```python
from build123d import *

# Parameters (mm, degrees)
SKETCH2_W           = 31.88
SKETCH2_H           = 23.87
BOSS_EXTRUDE1_DEPTH = 3.17
SKETCH3_R           = 2.455
BOSS_EXTRUDE2_DEPTH = 1.83
SHELL1_T            = -1.5
SKETCH4_R           = 3.24
SKETCH4_R_2         = 2.41
BOSS_EXTRUDE3_DEPTH = 1.47


with BuildPart() as part:
    # Sketch2 → Boss-Extrude1 (new body)
    with BuildSketch(Plane(origin=(0, 0, 0), x_dir=(1, 0, 0), z_dir=(0, 1, 0))):
        Rectangle(SKETCH2_W, SKETCH2_H)
    extrude(amount=-BOSS_EXTRUDE1_DEPTH)

    # Sketch3 → Boss-Extrude2 (add)
    with BuildSketch(Plane(origin=(0, 0, 0), x_dir=(1, 0, 0), z_dir=(0, 1, 0))):
        with Locations(Location((-12.135, 0, 0), (0, 0, 270))):
            Circle(SKETCH3_R)
        with Locations(Location((-4.045, 0, 0), (0, 0, 270))):
            Circle(SKETCH3_R)
        with Locations(Location((4.045, 0, 0), (0, 0, 270))):
            Circle(SKETCH3_R)
        with Locations(Location((12.135, 0, 0), (0, 0, 270))):
            Circle(SKETCH3_R)
    extrude(amount=BOSS_EXTRUDE2_DEPTH)

    # Shell1
    shell1_openings = [part.faces().sort_by_distance(p)[0] for p in [
        (0, -3.17, 0),
    ]]
    offset(amount=SHELL1_T, openings=shell1_openings, kind=Kind.INTERSECTION)

    # Sketch4 → Boss-Extrude3 (add)
    # profile 1 of 6: a face of its own
    with BuildSketch(Plane.XZ.offset(1.5)):
        with Locations(Location((-7.97, 3.978333333, 0), (0, 0, 90))):
            Circle(SKETCH4_R)
        with Locations(Location((-7.97, 3.978333333, 0), (0, 0, 90))):
            Circle(SKETCH4_R_2, mode=Mode.SUBTRACT)
    # profile 2 of 6: a face of its own
    with BuildSketch(Plane.XZ.offset(1.5)):
        with Locations(Location((0, 3.978333333, 0), (0, 0, 90))):
            Circle(SKETCH4_R)
        with Locations(Location((0, 3.978333333, 0), (0, 0, 90))):
            Circle(SKETCH4_R_2, mode=Mode.SUBTRACT)
    # profile 3 of 6: a face of its own
    with BuildSketch(Plane.XZ.offset(1.5)):
        with Locations(Location((7.97, 3.978333333, 0), (0, 0, 90))):
            Circle(SKETCH4_R)
        with Locations(Location((7.97, 3.978333333, 0), (0, 0, 90))):
            Circle(SKETCH4_R_2, mode=Mode.SUBTRACT)
    # profile 4 of 6: a face of its own
    with BuildSketch(Plane.XZ.offset(1.5)):
        with Locations(Location((0, -3.981666667, 0), (0, 0, 90))):
            Circle(SKETCH4_R)
        with Locations(Location((0, -3.981666667, 0), (0, 0, 90))):
            Circle(SKETCH4_R_2, mode=Mode.SUBTRACT)
    # profile 5 of 6: a face of its own
    with BuildSketch(Plane.XZ.offset(1.5)):
        with Locations(Location((7.97, -3.981666667, 0), (0, 0, 90))):
            Circle(SKETCH4_R)
        with Locations(Location((7.97, -3.981666667, 0), (0, 0, 90))):
            Circle(SKETCH4_R_2, mode=Mode.SUBTRACT)
    # profile 6 of 6: a face of its own
    with BuildSketch(Plane.XZ.offset(1.5)):
        with Locations(Location((-7.97, -3.981666667, 0), (0, 0, 90))):
            Circle(SKETCH4_R)
        with Locations(Location((-7.97, -3.981666667, 0), (0, 0, 90))):
            Circle(SKETCH4_R_2, mode=Mode.SUBTRACT)
    extrude(amount=BOSS_EXTRUDE3_DEPTH)


solid = part.part
```
Design review of the part built by this model. Coordinates are the model's own, in mm. A direction names the side the tool comes from. Give positions to 0.01 mm unless a question says otherwise; leave off trailing zeros. Order: outer loops, then holes, each group sorted by start corner. A loop starts at its lowest first (then second) coordinate and runs counter-clockwise, first axis right, second up. Notation, with made-up numbers: (33, 63.5) - (91, 63.5) arc R32 ccw to (91, 93.5) - close; hole circle Ø1 at (-6, 81). An arc over 180 degrees is marked (long way). Use a Markdown table: item, result. Add a question column.
(1) Machinability: for faces 1 (the face through (-14.44, -2, 0)), 2 (the face through (12, 1.83, 0)), which of the approach directions +Z, -Z, +X, -X, +Y, -Y give a long, thin tool a straight path to every point of the face, cutting with its end or side? Answer none if there is none.
(2) Add section A-A on y = -1.9. Give the number of separate pieces and of enclosed holes in the cut face, then the cut area to 3 significant figures.
(3) Add section D-D on z = 6.75. Give the boundary of the cut face in (x, y), then the cut area to 3 significant figures.
(4) Mouldability with a two-part tool opening along X and no side actions: class faces 3 (the face through (-4, 1.83, 0)), 4 (the face through (0, -1.5, -4)) as +X half, -X half, draft (parallel to the pull), parting line (faces both ways), or undercut.
(5) Add section B-B on z = -8. Give the boundary of the cut face in (x, y).
(6) Wall thickness on probe 1 along X at (y, z) = (-0.55, 0); probe 2 along X at (y, z) = (-1.6, -9.75); probe 3 along X at (y, z) = (1.45, -1.5): over which ranges is each line inside the solid? List them lowest first. Write a range as [from, to].
(7) Clearance check with flat-ended pins moving along their axes: P1, Ø2, axis at x = -12, z = -0.5, coming from the -Y side; P2, Ø0.6, axis at x = 12.5, z = -0.5, coming from the -Y side; P3, Ø4, axis at x = 0, z = 3.98, coming from the +Y side; P4, Ø1, axis at y = 1, z = -8.5, coming from the -X side. State where each tip first meets the part, or that it passes through.
(8) Add section C-C on x = 7.97. Give the boundary of the cut face in (y, z) (3 decimals), then the cut area to 3 significant figures.
Report:
| question | item | result |
|---|---|---|
| 1 | face 1 | -Y |
| 1 | face 2 | +Z, -Z, +X, -X, +Y |
| 2 | separate pieces | 7 |
| 2 | enclosed holes | 7 |
| 2 | area | 247 mm² |
| 3 | outline | (-15.94, -3.17) - (-14.44, -3.17) - (-14.44, -1.5) - (-9.65, -1.5) - (-9.65, -2.97) - (-6.29, -2.97) - (-6.29, -1.5) - (-1.68, -1.5) - (-1.68, -2.97) - (1.68, -2.97) - (1.68, -1.5) - (6.29, -1.5) - (6.29, -2.97) - (9.65, -2.97) - (9.65, -1.5) - (14.44, -1.5) - (14.44, -3.17) - (15.94, -3.17) - (15.94, 0) - (-15.94, 0) - close |
| 3 | area | 67.6 mm² |
| 4 | face 3 | draft |
| 4 | face 4 | undercut |
| 5 | outline | (-15.94, -3.17) - (-14.44, -3.17) - (-14.44, -1.5) - (14.44, -1.5) - (14.44, -3.17) - (15.94, -3.17) - (15.94, 0) - (-15.94, 0) - close |
| 6 | probe 1 | x = [-15.94, -13.09], [-11.18, -5], [-3.09, 3.09], [5, 11.18], [13.09, 15.94] |
| 6 | probe 2 | x = [-15.94, -14.44], [14.44, 15.94] |
| 6 | probe 3 | x = [-14.08, -10.19], [-5.99, -2.1], [2.1, 5.99], [10.19, 14.08] |
| 7 | P1 | stops at y = -1.5 |
| 7 | P2 | stops at y = 0.33 |
| 7 | P3 | stops at y = 0 |
| 7 | P4 | passes through |
| 8 | outline | (-3.17, -11.935) - (0, -11.935) - (0, 11.935) - (-3.17, 11.935) - (-3.17, 10.435) - (-1.5, 10.435) - (-1.5, 7.218) - (-2.97, 7.218) - (-2.97, 6.388) - (-1.5, 6.388) - (-1.5, 1.568) - (-2.97, 1.568) - (-2.97, 0.738) - (-1.5, 0.738) - (-1.5, -0.742) - (-2.97, -0.742) - (-2.97, -1.572) - (-1.5, -1.572) - (-1.5, -6.392) - (-2.97, -6.392) - (-2.97, -7.222) - (-1.5, -7.222) - (-1.5, -10.435) - (-3.17, -10.435) - close |
| 8 | area | 45.7 mm² |
